The model under review builds one solid part; all positions refer to its coordinate system, in mm. A direction names the side the tool comes from. Coordinates: 2 decimals unless noted, no trailing zeros. Order: outer loops, then holes, each group sorted by start corner. A loop starts at its lowest first (then second) coordinate and runs counter-clockwise, first axis right, second up. Notation, with made-up numbers: M 36,46.25 L 50,46.25 A32 cw 50,79.25 Z; hole C 55.5,39.25 d6. An arc over 180 degrees is marked long. Answer as CSV lines item,"result". Start each with the question number.
Q1. Wall thickness on L1, parallel to Z at x = 0, y = -6; L2, parallel to Z at x = 0, y = 0.5; L3, parallel to Z at x = -9.5, y = -9.5: over which ranges is each line inside the solid? List them lowest first. Write a range as [from, to].
Q2. Consider section B-B on z = -11. Write out the cut boundary in (x, y), and give its area (3 significant figures).
Q3. The part is to be moulded in two halves that separate along Z. For faces 1 (the face through (6.86, 0.23, 6.59)), 2 (the face through (4.699, -33.64, -4.715)), 3 (the face through (0, -33, 5)), 4 (the face through (-5, -33, 0)), say which applies: +Z half, -Z half, draft (parallel to the pull), parting line (faces both ways), or undercut.
Q4. Consider section C-C on x = 11. Write out the cut boundary in (y, z).
Q5. Machinability: for faces 5 (the face through (-4.699, -33.64, 4.715)), 6 (the face through (-4.715, -33.64, -4.699)), 7 (the face through (4.88, -0.96, 1.08)), 8 (the face through (8.56, -9.39, -0.54)), which of the approach directions +Z, -Z, +X, -X, +Y, -Y give a long, thin tool a straight path to every point of the face, cutting with its end or side? Answer none if there is none.
Q6. Consider section D-D on y = -7.5. State how many separate pieces and enclosed holes the cut face has, and give its area (3 significant figures).
Q7. Consider section A-A on y = -33.5. Write out the cut boundary in (x, z), and give its area (3 significant figures).
Q8. For P1, Ø1, axis at y = -3.5, z = -3.5, coming from the +X side; P2, Ø4, axis at x = 8, z = -7.5, coming from the -Y side; P3, Ø8, axis at x = 7.78, z = 7.78, coming from the -Y side, all flat-tipped, find the tip position at first contact; note any pin that passes through.
Solid Edge part; units mm, degrees
sketch "Sketch1" plane through (0, 0, 0) normal (0, -1, 0) x (1, 0, 0)
  circle A0 centre (0, 0) radius 16.5
extrude "Protrusion1" add sketch "Sketch1" against normal blind 2
sketch "Sketch2" plane through (0, 0, 0) normal (0, -1, 0) x (1, 0, 0)
  circle A0 centre (0, 0) radius 15
extrude "ProtrusiónExtruida_2" add sketch "Sketch2" along normal blind 17.5
sketch "Sketch3" plane through (0, -17.5, 0) normal (0, -1, 0) x (1, 0, 0)
  circle A0 centre (0, 0) radius 7.5
extrude "ProtrusiónExtruida_3" add sketch "Sketch3" along normal blind 6
sketch "Sketch4" plane through (0, -23.5, 0) normal (0, -1, 0) x (1, 0, 0)
  line L0 (5, -5) -> (-5, -5)
  line L1 (-5, -5) -> (-5, 5)
  line L2 (-5, 5) -> (5, 5)
  line L3 (5, 5) -> (5, -5)
  dimension "D1" = 5
  dimension "D2" = 5
extrude "ProtrusiónExtruida_4" add sketch "Sketch4" along normal blind 20
hole "Agujero_1" at (-11, -17.5, 0) direction (0, 1, 0) diameter 3 end up to next counterbore diameter 5 counterbore depth 16
pattern_circular "Pattern1" count 8 over 360 about axis through (0, -17.5, 0) along (0, 1, 0) of "Agujero_1"
sketch "Sketch5" plane through (0, 2, 0) normal (0, 1, 0) x (0, 0, -1)
  circle A0 centre (0, 0) radius 5
extrude "VaciadoExtruido_1" cut sketch "Sketch5" against normal blind 6
fillet "Redondeo_1" radius 1 4 edges at (-5, -33.5, -5) (-5, -33.5, 5) (5, -33.5, 5) (5, -33.5, -5)
hole "Agujero_9" at (0, -43.5, 0) direction (0, 1, 0) diameter 4.917 depth 18 tip angle 118 thread major 6 thread length 15
properties part number "1976-1100-014" material "Aluminio, 7075-T6"
Evaluation:
1,L1,"z = [-15, -13.5], [-8.5, 8.5], [13.5, 15]"
1,L2,"z = [-16.5, -12.5], [-9.5, -5], [5, 9.5], [12.5, 16.5]"
1,L3,"z = [-11.61, -9.59], [-5.97, -2], [2, 5.97], [9.59, 11.61]"
2,outline,"M -12.3,0 L -10.2,0 L -10.2,-17.5 L -2.5,-17.5 L -2.5,-1.5 L -1.5,-1.5 L -1.5,2 L -12.3,2 Z; M 1.5,-1.5 L 2.5,-1.5 L 2.5,-17.5 L 10.2,-17.5 L 10.2,0 L 12.3,0 L 12.3,2 L 1.5,2 Z"
2,area,"316 mm²"
3,face 1,"undercut"
3,face 2,"-Z half"
3,face 3,"+Z half"
3,face 4,"draft"
4,outline,"M -17.5,-10.2 L 0,-10.2 L 0,-12.3 L 2,-12.3 L 2,-1.5 L -1.5,-1.5 L -1.5,-2.5 L -17.5,-2.5 Z; M -17.5,2.5 L -1.5,2.5 L -1.5,1.5 L 2,1.5 L 2,12.3 L 0,12.3 L 0,10.2 L -17.5,10.2 Z"
5,face 5,"+Z, -X, -Y"
5,face 6,"-Z, -X, -Y"
5,face 7,"+Y"
5,face 8,"-Y"
6,separate pieces,"1"
6,enclosed holes,"8"
6,area,"550 mm²"
7,outline,"M -5,-4 A1 ccw -4,-5 L 4,-5 A1 ccw 5,-4 L 5,4 A1 ccw 4,5 L -4,5 A1 ccw -5,4 Z; hole C 0,0 d4.92"
7,area,"80.2 mm²"
8,P1,"stops at x = 14.7"
8,P2,"stops at y = -1.5"
8,P3,"stops at y = -23.5"
